```python
from build123d import *

# Parameters (mm, degrees)
F0_R     = 20.32
F1_DEPTH = 9.271
F2_R     = 1.5875
F3_DEPTH = 60.511199891
F4_R     = 6.35


# Not quite as in the source:
# - a feature names something its author has since deleted; it is built from what else it names


with BuildPart() as f1:
    # F0 (on Top) → F1 (new body)
    with BuildSketch(Plane.XY):
        with BuildLine():
            ThreePointArc((23.9050999455, -6.4692674698), (24.5490837421, -3.2630832697), (24.765, 0))
            ThreePointArc((24.765, 0), (19.6285885254, 15.1004548773), (6.35, 23.9370575677))
            ThreePointArc((6.35, 23.9370575677), (4.0651088886, 24.4290833787), (1.7440091422, 24.703515076))
            ThreePointArc((1.7440091422, 24.703515076), (1.8643178935, 24.3286489263), (1.905, 23.9370575677))
            ThreePointArc((1.905, 23.9370575677), (-0.3915913586, 22.0727396742), (-1.7440091422, 24.703515076))
            ThreePointArc((-1.7440091422, 24.703515076), (-4.0651088886, 24.4290833787), (-6.35, 23.9370575677))
            ThreePointArc((-6.35, 23.9370575677), (-21.4471191247, 12.3825), (-23.9050999455, -6.4692674698))
            ThreePointArc((-23.9050999455, -6.4692674698), (-23.1887612414, -8.6940541227), (-22.2658761897, -10.8414013165))
            ThreePointArc((-22.2658761897, -10.8414013165), (-20.1370690632, -10.1581864481), (-18.8250999455, -11.9685287839))
            ThreePointArc((-18.8250999455, -11.9685287839), (-19.3113489683, -13.239815795), (-20.5218670475, -13.8621137596))
            ThreePointArc((-20.5218670475, -13.8621137596), (-19.1236523528, -15.735029256), (-17.5550999455, -17.4677900979))
            ThreePointArc((-17.5550999455, -17.4677900979), (0, -24.765), (17.5550999455, -17.4677900979))
            ThreePointArc((17.5550999455, -17.4677900979), (19.1236523528, -15.735029256), (20.5218670475, -13.8621137596))
            ThreePointArc((20.5218670475, -13.8621137596), (19.0803215513, -11.0160287839), (22.2658761897, -10.8414013165))
            ThreePointArc((22.2658761897, -10.8414013165), (23.1887612414, -8.6940541227), (23.9050999455, -6.4692674698))
        make_face()
        Circle(F0_R, mode=Mode.SUBTRACT)
        with BuildLine():
            ThreePointArc((-22.2658761897, -10.8414013165), (-23.1887612414, -8.6940541227), (-23.9050999455, -6.4692674698))
            ThreePointArc((-23.9050999455, -6.4692674698), (-26.2293612595, -15.1435287839), (-17.5550999455, -17.4677900979))
            ThreePointArc((-17.5550999455, -17.4677900979), (-19.1236523528, -15.735029256), (-20.5218670475, -13.8621137596))
            ThreePointArc((-20.5218670475, -13.8621137596), (-22.3798783397, -12.9210287839), (-22.2658761897, -10.8414013165))
        make_face()
        with BuildLine():
            ThreePointArc((17.5550999455, -17.4677900979), (26.2293612595, -15.1435287839), (23.9050999455, -6.4692674698))
            ThreePointArc((23.9050999455, -6.4692674698), (23.1887612414, -8.6940541227), (22.2658761897, -10.8414013165))
            ThreePointArc((22.2658761897, -10.8414013165), (22.5404422812, -11.3754979015), (22.6350999455, -11.9685287839))
            ThreePointArc((22.6350999455, -11.9685287839), (22.0013869566, -13.3872797611), (20.5218670475, -13.8621137596))
            ThreePointArc((20.5218670475, -13.8621137596), (19.1236523528, -15.735029256), (17.5550999455, -17.4677900979))
        make_face()
        with BuildLine():
            Line((30.2550999455, -7.9427900979), (23.9050999455, -6.4692674698))
            ThreePointArc((23.9050999455, -6.4692674698), (26.2293612595, -15.1435287839), (17.5550999455, -17.4677900979))
            ThreePointArc((17.5550999455, -17.4677900979), (0, -24.765), (-17.5550999455, -17.4677900979))
            ThreePointArc((-17.5550999455, -17.4677900979), (-26.2293612595, -15.1435287839), (-23.9050999455, -6.4692674698))
            Line((-23.9050999455, -6.4692674698), (-30.2550999455, -7.9427900979))
            Line((-30.2550999455, -7.9427900979), (-30.2550999455, -33.3427900979))
            Line((-30.2550999455, -33.3427900979), (30.2550999455, -33.3427900979))
            Line((30.2550999455, -33.3427900979), (30.2550999455, -7.9427900979))
        make_face()
        with BuildLine():
            ThreePointArc((1.7440091422, 24.703515076), (4.0651088886, 24.4290833787), (6.35, 23.9370575677))
            ThreePointArc((6.35, 23.9370575677), (0, 30.2870575677), (-6.35, 23.9370575677))
            ThreePointArc((-6.35, 23.9370575677), (-4.0651088886, 24.4290833787), (-1.7440091422, 24.703515076))
            ThreePointArc((-1.7440091422, 24.703515076), (0, 25.8420575677), (1.7440091422, 24.703515076))
        make_face()
    extrude(amount=F1_DEPTH)

    # F2 (on face) → F3 (cut, through all)
    with BuildSketch(Plane.YZ.offset(30.2550999455)):
        with Locations((-28.5802900979, 4.7625)):
            Circle(F2_R)
        with Locations((-22.2315602249, 4.6355)):
            Circle(F2_R)
    extrude(amount=-F3_DEPTH, mode=Mode.SUBTRACT)

    # F4
    f4_edges = [f1.edges().sort_by_distance(p)[0] for p in [
        (-23.9051, -6.469267, 4.6355),
        (23.9051, -6.469267, 4.6355),
        (6.35, 23.937058, 4.6355),
        (-6.35, 23.937058, 4.6355),
    ]]
    fillet(f4_edges, radius=F4_R)


solid = f1.part
```
The model under review builds one solid part; all positions refer to its coordinate system, in mm. Round coordinates to 2 decimals unless told otherwise and drop trailing zeros. Order: outer loops, then holes, each group sorted by start corner. A loop starts at its lowest first (then second) coordinate and runs counter-clockwise, first axis right, second up. Notation, with made-up numbers: (61, 60.25) - (97, 60.25) arc R23 cw to (97, 77.25) - close; hole circle Ø6 at (59, 18.5). An arc over 180 degrees is marked (long way). Answer in a Markdown table with one row per item.
(1) Take a section at C-C on y = -6.5. Write out the cut boundary in (x, z).
Result set:
| item | result |
|---|---|
| outline | (-27.02, 0) - (-19.25, 0) - (-19.25, 9.27) - (-27.02, 9.27) - close; (19.25, 0) - (27.02, 0) - (27.02, 9.27) - (19.25, 9.27) - close |
(2) Clearance check with flat-ended pins moving along their axes: P1, Ø2, axis at y = 5.5, z = 4, coming from the -X side; P2, Ø2, axis at x = 6.5, z = 1.5, coming from the +Y side. State where each tip first meets the part, or that it passes through.
Result set:
| item | result |
|---|---|
| P1 | stops at x = -24.35 |
| P2 | stops at y = 27.11 |
(3) For line 1 (X direction, y = -10.5, z = 0.5); line 2 (Y direction, x = 5, z = 4.5); line 3 (Y direction, x = -15.5, z = 5), list the stretches that pass through material, from the lowest coordinate up. Write a range as from..to.
Result set:
| item | result |
|---|---|
| line 1 | x = -30.26..-21.94, -19.52..-17.4, 17.4..19.52, 21.94..30.26 |
| line 2 | y = -33.34..-30.15, -27.01..-23.81, -20.65..-19.7, 19.7..27.85 |
| line 3 | y = -33.34..-30.15, -27.01..-23.78, -20.69..-13.14, 13.14..19.31 |
(4) Take a section at A-A on x = 0. Write out the cut boundary in (y, z) (1 decimal), plus the area to 3 significant figures.
Result set:
| item | result |
|---|---|
| outline | (-33.3, 0) - (-20.3, 0) - (-20.3, 9.3) - (-33.3, 9.3) - close; (20.3, 0) - (22, 0) - (22, 9.3) - (20.3, 9.3) - close; (25.8, 0) - (30.3, 0) - (30.3, 9.3) - (25.8, 9.3) - close; hole circle Ø3.2 at (-28.6, 4.8); hole circle Ø3.2 at (-22.2, 4.6) |
| area | 162 mm2 |
(5) Mouldability with a two-part tool opening along Z and no side actions: class faces 1 (the face through (0, -33.343, 5)), 2 (the face through (0.424, -30.166, 4.832)), 3 (the face through (0, -22, 9.271)) as released by +Z, released by -Z, zero draft, split by the parting line, or undercut.
Result set:
| item | result |
|---|---|
| face 1 | zero draft |
| face 2 | undercut |
| face 3 | released by +Z |
(6) Take a section at D-D on z = 1.5. Count the separate pieces of the cut face and the enclosed holes in it, plus the area to 3 significant figures.
Result set:
| item | result |
|---|---|
| separate pieces | 1 |
| enclosed holes | 4 |
| area | 1,640 mm2 |
(7) Take a section at B-B on y = 6.5. Write out the cut boundary in (x, z), plus the area to 3 significant figures.
Result set:
| item | result |
|---|---|
| outline | (-23.9, 0) - (-19.25, 0) - (-19.25, 9.27) - (-23.9, 9.27) - close; (19.25, 0) - (23.9, 0) - (23.9, 9.27) - (19.25, 9.27) - close |
| area | 86.1 mm2 |
